```python
from build123d import *

# Parameters (mm, degrees)
SKETCH1_W           = 80
SKETCH1_H           = 82.3
BOSS_EXTRUDE1_DEPTH = 55
CUT_EXTRUDE1_DEPTH  = 50
SKETCH3_R           = 1.65
CUT_EXTRUDE2_DEPTH  = 25
SKETCH4_W           = 15
SKETCH4_H           = 27
SKETCH4_W_2         = 24
SKETCH4_H_2         = 20
CUT_EXTRUDE3_DEPTH  = 20
SKETCH6_R           = 6.5
CUT_EXTRUDE4_DEPTH  = 20
SKETCH7_W           = 3
SKETCH7_H           = 3
BOSS_EXTRUDE2_DEPTH = 30
SKETCH8_R           = 1.65
CUT_EXTRUDE5_DEPTH  = 25


with BuildPart() as part:
    # Sketch1 → Boss-Extrude1 (new body)
    with BuildSketch(Plane.XY):
        with Locations((40, 41.15)):
            Rectangle(SKETCH1_W, SKETCH1_H)
    extrude(amount=BOSS_EXTRUDE1_DEPTH)

    # Sketch2 → Cut-Extrude1 (cut)
    with BuildSketch(Plane.XY.offset(55)):
        Polygon((80, 5), (80, 77.3), (8, 77.3), (8, 74.3), (5, 74.3), (5, 8), (8, 8), (8, 5), align=None)
    extrude(amount=-CUT_EXTRUDE1_DEPTH, mode=Mode.SUBTRACT)

    # Sketch3 → Cut-Extrude2 (cut)
    with BuildSketch(Plane.XY.offset(55)):
        with Locations((4, 78.3)):
            Circle(SKETCH3_R)
        with Locations((4, 4)):
            Circle(SKETCH3_R)
    extrude(amount=-CUT_EXTRUDE2_DEPTH, mode=Mode.SUBTRACT)

    # Sketch4 → Cut-Extrude3 (cut)
    with BuildSketch(Plane.XY.offset(5)):
        with Locations((18, 41.15)):
            Rectangle(SKETCH4_W, SKETCH4_H)
        with Locations((68, 17)):
            Rectangle(SKETCH4_W_2, SKETCH4_H_2)
    extrude(amount=-CUT_EXTRUDE3_DEPTH, mode=Mode.SUBTRACT)

    # Sketch6 → Cut-Extrude4 (cut)
    with BuildSketch(Plane.XZ.offset(-77.3)):
        with Locations((65, 20.5)):
            Circle(SKETCH6_R)
    extrude(amount=-CUT_EXTRUDE4_DEPTH, mode=Mode.SUBTRACT)

    # Sketch7 → Boss-Extrude2 (add)
    with BuildSketch(Plane(origin=(80, 0, 0), x_dir=(0, 0, -1), z_dir=(1, 0, 0))):
        with Locations((-6.5, 75.8)):
            Rectangle(SKETCH7_W, SKETCH7_H)
    extrude(amount=-BOSS_EXTRUDE2_DEPTH)

    # Sketch8 → Cut-Extrude5 (cut)
    with BuildSketch(Plane(origin=(80, 0, 0), x_dir=(0, 0, -1), z_dir=(1, 0, 0))):
        with Locations((-4.004640203, 78.3)):
            Circle(SKETCH8_R)
    extrude(amount=-CUT_EXTRUDE5_DEPTH, mode=Mode.SUBTRACT)


solid = part.part
```
Verification items for the finished model (mm, model axes). A direction names the side the tool comes from. Round coordinates to 2 decimals unless told otherwise and drop trailing zeros. Write each loop counter-clockwise with the first axis right and the second up, starting at its lowest first coordinate (ties: lowest second). Pieces come first, ordered by that corner, then holes.
1. Section check D-D on x = 22.5. Enter the section's corners in (y, z), plus the area to 4 significant figures.
2. Access from +Z, -Z, +X, -X, +Y, -Y to the whole of each face (thin tool, end or side, straight path). Record for faces 4 (the flat face through (65, 76, 8)), 5 (the cylindrical face through (71.2, 79.76, 22.45)), 6 (the flat face through (18, 54.65, 3)).
3. Section check A-A on x = 73. Enter the section's corners in (y, z).
4. Section check B-B on x = 65. Enter the section's corners in (y, z).
5. Gauge pin test, flat ends, axial feed: P1, Ø1.5, axis at y = 6, z = 41.5, coming from the +X side; P2, Ø8, axis at y = 62, z = 31.5, coming from the +X side; P3, Ø6, axis at x = 14, y = 50, coming from the -Z side; P4, Ø3, axis at y = 78.3, z = 4, coming from the +X side. Record the tip position at first contact, or that the pin passes through.
6. Section check C-C on z = 20.5. Enter the section's corners in (x, y), plus the area to 3 significant figures.
7. Scan lines: L1, parallel to Y at x = 4, z = 49; L2, parallel to Y at x = 31, z = 21; L3, parallel to X at y = 78.3, z = 45.5. Record each from-to range of solid material in increasing order.
8. Draft check along Y on faces 1 (the flat face through (80, 3, 27)), 2 (the flat face through (39, 0, 27)), 3 (the cylindrical face through (2.69, 3, 42.68)). Enter one of: +Y half, -Y half, draft (parallel to the pull), parting line (faces both ways), or undercut.
Answer:
1. outline: (0, 0) - (27.65, 0) - (27.65, 5) - (5, 5) - (5, 55) - (0, 55) - close; (54.65, 0) - (82.3, 0) - (82.3, 55) - (77.3, 55) - (77.3, 5) - (54.65, 5) - close
1. area: 776.5 mm2
2. face 4: +Z, +X
2. face 5: +Y
2. face 6: +Z, -Z
3. outline: (0, 0) - (7, 0) - (7, 5) - (5, 5) - (5, 55) - (0, 55) - close; (27, 0) - (82.3, 0) - (82.3, 55) - (77.3, 55) - (77.3, 8) - (74.3, 8) - (74.3, 5) - (27, 5) - close; hole circle Ø3.3 at (78.3, 4)
4. outline: (0, 0) - (7, 0) - (7, 5) - (5, 5) - (5, 55) - (0, 55) - close; (27, 0) - (82.3, 0) - (82.3, 14) - (77.3, 14) - (77.3, 8) - (74.3, 8) - (74.3, 5) - (27, 5) - close; (77.3, 27) - (82.3, 27) - (82.3, 55) - (77.3, 55) - close; hole circle Ø3.3 at (78.3, 4)
5. P1: stops at x = 8
5. P2: stops at x = 5
5. P3: passes through
5. P4: stops at x = 55
6. outline: (0, 0) - (80, 0) - (80, 5) - (8, 5) - (8, 8) - (5, 8) - (5, 74.3) - (8, 74.3) - (8, 77.3) - (58.5, 77.3) - (58.5, 82.3) - (0, 82.3) - close; (71.5, 77.3) - (80, 77.3) - (80, 82.3) - (71.5, 82.3) - close
6. area: 1,110 mm2
7. L1: y = 0 to 2.35, 5.65 to 76.65, 79.95 to 82.3
7. L2: y = 0 to 5, 77.3 to 82.3
7. L3: x = 0 to 2.35, 5.65 to 80
8. face 1: draft
8. face 2: -Y half
8. face 3: undercut
